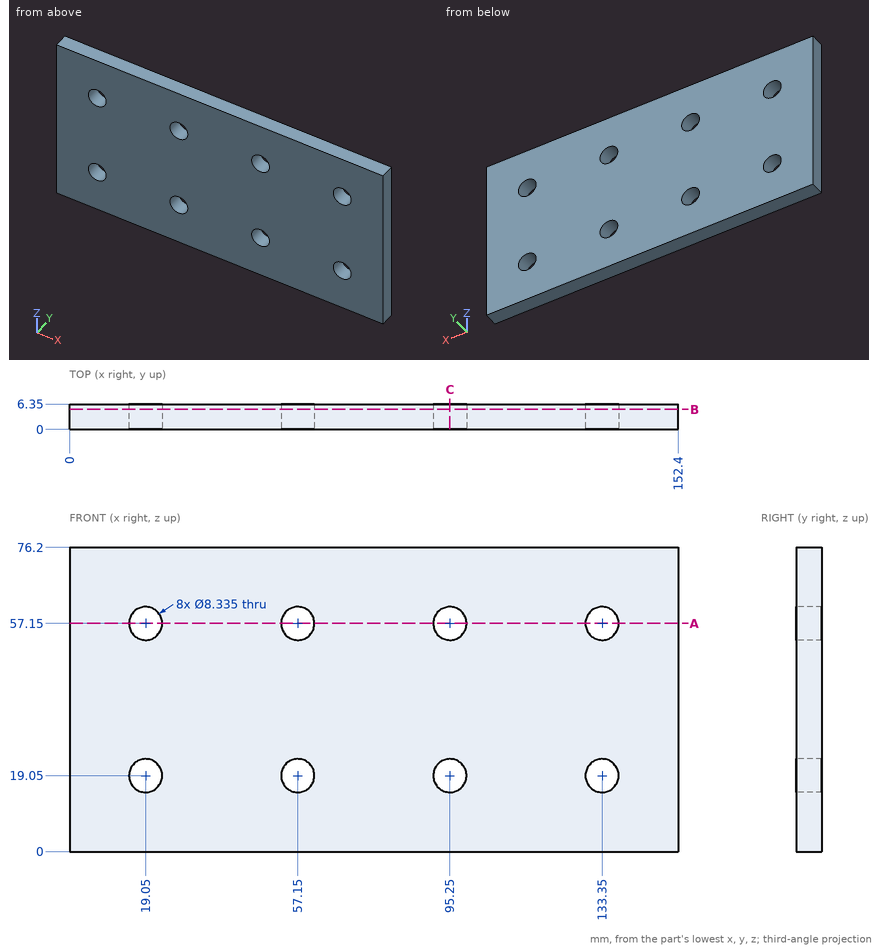
Can you work these out from the drawing? Everything is in mm from the part's minimum corner. Round coordinates to 2 decimals unless told otherwise and drop trailing zeros. Loops run counter-clockwise (first coordinate to the right, second up) from the corner with the lowest first, then second, coordinate; pieces in that order, holes last. Notation, with made-up numbers: (86.5, -32) - (115.5, -32) arc R32 cw to (115.5, -6) - close; hole circle Ø9 at (-19.5, 86.5). An arc over 180 degrees is marked (long way). Answer in a Markdown table with one row per item. Add a question column.
(1) If we section it at A-A (z = 57.15): Please give me the cut outline in (x, y).
(2) If we section it at B-B (y = 5): State how many separate pieces and enclosed holes the cut face has, plus the area to 3 significant figures.
(3) I need wall thicknesses on line 1 along Z through (x, y) = (95.25, 3.5); line 2 along Z through (x, y) = (93, 4.5); line 3 along X through (y, z) = (2, 58). Which ranges of each line are inside material? Lowest first, please.
(4) If we section it at C-C (x = 95.25): Please give me the cut outline in (y, z), plus the area to 3 significant figures.
Model answer:
| question | item | result |
|---|---|---|
| 1 | outline | (0, 0) - (14.88, 0) - (14.88, 6.35) - (0, 6.35) - close; (23.22, 0) - (52.98, 0) - (52.98, 6.35) - (23.22, 6.35) - close; (61.32, 0) - (91.08, 0) - (91.08, 6.35) - (61.32, 6.35) - close; (99.42, 0) - (129.18, 0) - (129.18, 6.35) - (99.42, 6.35) - close; (137.52, 0) - (152.4, 0) - (152.4, 6.35) - (137.52, 6.35) - close |
| 2 | separate pieces | 1 |
| 2 | enclosed holes | 8 |
| 2 | area | 11,200 mm² |
| 3 | line 1 | z = 0 to 14.88, 23.22 to 52.98, 61.32 to 76.2 |
| 3 | line 2 | z = 0 to 15.54, 22.56 to 53.64, 60.66 to 76.2 |
| 3 | line 3 | x = 0 to 14.97, 23.13 to 53.07, 61.23 to 91.17, 99.33 to 129.27, 137.43 to 152.4 |
| 4 | outline | (0, 0) - (6.35, 0) - (6.35, 14.88) - (0, 14.88) - close; (0, 23.22) - (6.35, 23.22) - (6.35, 52.98) - (0, 52.98) - close; (0, 61.32) - (6.35, 61.32) - (6.35, 76.2) - (0, 76.2) - close |
| 4 | area | 378 mm² |
